```python
from build123d import *

# Parameters (mm, degrees)
SKETCH1_W          = 50.8
SKETCH1_H          = 44.45
EXTRUDE1_DEPTH     = 57.023
SKETCH5_R          = 17.4625
EXTRUDE2_DEPTH     = 5.969
SKETCH6_W          = 10.31875
SKETCH6_H          = 14.478
CUT_EXTRUDE4_DEPTH = 30.48
HOLE1_D            = 7.1374
HOLE1_DEPTH        = 57.023
HOLE2_D            = 8.7376
HOLE2_DEPTH        = 44.45


with BuildPart() as part:
    # Sketch1 → Extrude1 (new body)
    with BuildSketch(Plane(origin=(0, 0, 0), x_dir=(0, 0, -1), z_dir=(1, 0, 0))):
        Rectangle(SKETCH1_W, SKETCH1_H)
    extrude(amount=EXTRUDE1_DEPTH)

    # S2D0002 → Cut-Revolve1 (revolve, cut)
    with BuildSketch(Plane(origin=(0, 14.3002, 0), x_dir=(-1, 0, 0), z_dir=(0, 1, 0)), mode=Mode.PRIVATE) as cut_revolve1_sk:
        Polygon((-18.8849, -25.146), (-22.225, -25.146), (-22.225, -25.4), (-12.7, -25.4), (-12.7, -11.176), (-17.6784, -11.176), (-17.6784, -21.929393135), (-18.342306865, -22.5933), align=None)
    revolve(cut_revolve1_sk.sketch.rotate(Axis((12.7, 14.3002, -19.13842003), (0, 0, 1)), 180), axis=Axis((12.7, 14.3002, -19.13842003), (0, 0, 1)), mode=Mode.SUBTRACT)  # turned: the seam where the file's is

    # Sketch3 → Cut-Revolve2 (revolve, cut)
    with BuildSketch(Plane(origin=(41.148, 0, -25.146), x_dir=(1, 0, 0), z_dir=(0, 1, 0))):
        Polygon((6.1849, 0), (9.525, 0), (9.525, 0.254), (0, 0.254), (0, -13.97), (4.9784, -13.97), (4.9784, -3.216606865), (5.642306865, -2.5527), align=None)
    revolve(axis=Axis((41.148, 0, -3.189624441), (0, 0, -1)), mode=Mode.SUBTRACT)

    # Sketch4 → Cut-Revolve3 (revolve, cut)
    with BuildSketch(Plane(origin=(53.975, 0, 0), x_dir=(0, -1, 0), z_dir=(0, 0, 1)), mode=Mode.PRIVATE) as cut_revolve3_sk:
        Polygon((6.1849, 0), (9.525, 0), (9.525, 3.048), (0, 3.048), (0, -11.3538), (4.9784, -11.3538), (4.9784, -3.216606865), (5.642306865, -2.5527), align=None)
    revolve(cut_revolve3_sk.sketch.rotate(Axis((38.879609832, 0, 0), (1, 0, 0)), 270), axis=Axis((38.879609832, 0, 0), (1, 0, 0)), mode=Mode.SUBTRACT)  # turned: the seam where the file's is

    # Sketch5 → Extrude2 (add)
    with BuildSketch(Plane.ZY):
        Circle(SKETCH5_R)
    extrude(amount=EXTRUDE2_DEPTH)

    # Sketch6 → Revolve1 (revolve)
    with BuildSketch(Plane(origin=(0, 0, 0), x_dir=(0, 0, 1), z_dir=(0, -1, 0)), mode=Mode.PRIVATE) as revolve1_sk:
        with Locations((-5.159375, 13.208)):
            Rectangle(SKETCH6_W, SKETCH6_H)
    revolve(revolve1_sk.sketch.rotate(Axis((5.754582971, 0, 0), (-1, 0, 0)), 180), axis=Axis((5.754582971, 0, 0), (-1, 0, 0)))  # turned: the seam where the file's is

    # S2D0001 → Cut-Revolve4 (revolve, cut)
    with BuildSketch(Plane(origin=(-18.511260017, 3.2639, 0), x_dir=(0, 1, 0), z_dir=(0, 0, 1)), mode=Mode.PRIVATE) as cut_revolve4_sk:
        Polygon((0, 0), (0, -14.650460017), (-3.2639, -14.650460017), (-3.2639, 1.935739983), (1.1176, 1.935739983), align=None)
    revolve(cut_revolve4_sk.sketch.rotate(Axis((0, 0, 0), (-1, 0, 0)), 270), axis=Axis((0, 0, 0), (-1, 0, 0)), mode=Mode.SUBTRACT)  # turned: the seam where the file's is

    # Sketch8 → Cut-Revolve5 (revolve, cut)
    with BuildSketch(Plane(origin=(0, 0, 0), x_dir=(0, 0, -1), z_dir=(0, 1, 0)), mode=Mode.PRIVATE) as cut_revolve5_sk:
        with BuildLine():
            Line((-10.31875, 13.0302), (-10.033, 13.7922))
            Line((-10.033, 13.7922), (-10.033, 19.431))
            ThreePointArc((-10.033, 19.431), (-9.932678675, 19.974796865), (-9.644922533, 20.447))
            Line((-9.644922533, 20.447), (-10.31875, 20.447))
            Line((-10.31875, 20.447), (-10.31875, 13.0302))
        make_face()
    revolve(cut_revolve5_sk.sketch.rotate(Axis((-12.65936, 0, 0), (-1, 0, 0)), 180), axis=Axis((-12.65936, 0, 0), (-1, 0, 0)), mode=Mode.SUBTRACT)  # turned: the seam where the file's is

    # Sketch12 → Cut-Extrude4 (cut, symmetric)
    with BuildSketch(Plane(origin=(0, 0, 0), x_dir=(0, -1, 0), z_dir=(0, 0, -1))):
        Polygon((8.5852, 20.447), (8.5852, 15.494), (10.033, 14.0462), (10.033, 20.447), align=None)
        Polygon((-8.5852, 20.447), (-8.5852, 15.494), (-10.033, 14.0462), (-10.033, 20.447), align=None)
    extrude(amount=CUT_EXTRUDE4_DEPTH, both=True, mode=Mode.SUBTRACT)

    # Hole1
    with Locations(Plane.ZY):
        with Locations((-19.05, -15.875), (19.05, 15.875)):
            Hole(HOLE1_D / 2, depth=HOLE1_DEPTH)

    # Hole2
    with Locations(Plane(origin=(0, 22.225, 0), x_dir=(-1, 0, 0), z_dir=(0, 1, 0))):
        with Locations((-26.797, -19.05), (-26.797, 19.05)):
            Hole(HOLE2_D / 2, depth=HOLE2_DEPTH)


solid = part.part
```
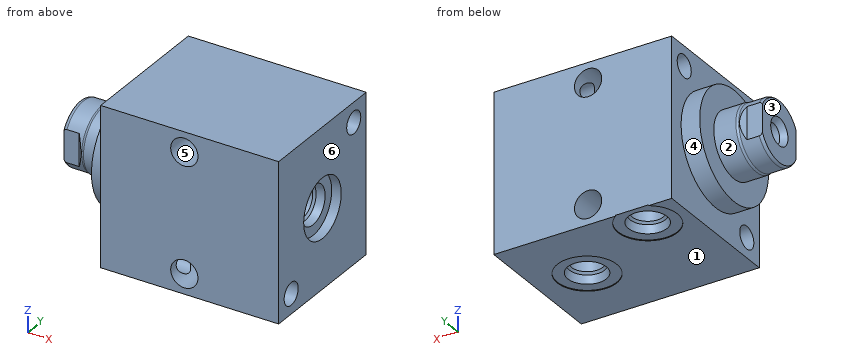
Source: CAD feature listing. Evaluate the final solid. Frame: model axes, mm. Face numbers are marked on the shaded views. A direction names the side the tool comes from. Round coordinates to 2 decimals unless told otherwise and drop trailing zeros. Loops run counter-clockwise (first coordinate to the right, second up) from the corner with the lowest first, then second, coordinate; pieces in that order, holes last. Notation, with made-up numbers: M -32,-7 L -27,-7 A18 cw -27,4 Z; hole C 61.25,51.25 d4. An arc over 180 degrees is marked long. Use a Markdown table: item, result. Add a question column.
1. Line query: line 1 (Z direction, x = 27, y = 7); line 2 (Y direction, x = -12, z = 0); line 3 (X direction, y = -11, z = 19). Output: solid intervals per line, ascending.
2. Section query C-C on x = -10.5. Return the cut outline in (y, z).
3. Mould query, pull axis X, two halves, no side actions, for the marked faces 3, 4, 5 and 6. Classes: pulls with the +X half, pulls with the -X half, needs draft (parallel to the pull), parting line crosses it, or undercut.
4. Section query B-B on x = 12.7. Give the number of separate pieces and of enclosed holes in the cut face, then the cut area to 3 significant figures.
5. Reachability of the marked faces 1 and 2 from +Z, -Z, +X, -X, +Y, -Y: full face, straight path, thin tool, end or side. Return the list, or none.
6. Section query A-A on z = 19.05. Return the cut outline in (x, y) (3 decimals), then the cut area to 3 significant figures.
7. Contact query for flat-ended pins moving along their axis: P1, Ø2, axis at y = 0.5, z = 1.5, coming from the -X side; P2, Ø1, axis at y = -8, z = 10, coming from the -X side; P3, Ø5.5, axis at x = -18, z = -1.5, coming from the +Y side; P4, Ø9.5, axis at y = -2.5, z = -4.5, coming from the +X side. Output: stop coordinate, or through.
Reported:
| question | item | result |
|---|---|---|
| 1 | line 1 | z = -25.4 to -23.41, -14.69 to 14.69, 23.41 to 25.4 |
| 1 | line 2 | y = -10.32 to -3.26, 3.26 to 10.32 |
| 1 | line 3 | x = 0 to 22.43, 31.17 to 57.02 |
| 2 | outline | C 0,0 d20.64; hole C 0,0 d6.53 |
| 3 | face 3 | pulls with the -X half |
| 3 | face 4 | needs draft |
| 3 | face 5 | undercut |
| 3 | face 6 | pulls with the +X half |
| 4 | separate pieces | 1 |
| 4 | enclosed holes | 2 |
| 4 | area | 2,030 mm² |
| 5 | face 1 | -Z, +X, -X, +Y, -Y |
| 5 | face 2 | -X |
| 6 | outline | M 0,-22.225 L 22.428,-22.225 L 22.428,12.306 L 0,12.306 Z; M 0,19.444 L 22.428,19.444 L 22.428,22.225 L 0,22.225 Z; M 31.166,-22.225 L 57.023,-22.225 L 57.023,12.306 L 31.166,12.306 Z; M 31.166,19.444 L 57.023,19.444 L 57.023,22.225 L 31.166,22.225 Z |
| 6 | area | 1,800 mm² |
| 7 | P1 | stops at x = -3.86 |
| 7 | P2 | stops at x = -5.97 |
| 7 | P3 | stops at y = 8.83 |
| 7 | P4 | stops at x = 57.02 |
